Part model, mm, in its own coordinate system. Give positions to 0.01 mm unless a question says otherwise; leave off trailing zeros. Write each loop counter-clockwise with the first axis right and the second up, starting at its lowest first coordinate (ties: lowest second). Pieces come first, ordered by that corner, then holes.
```python
from build123d import *

# Parameters (mm, degrees)
F3_DEPTH = 13.0048
F4_D     = 15
F5_D     = 12
F6_D     = 27.94


with BuildPart() as f3:
    # F2 (on Top) → F3 (new body)
    with BuildSketch(Plane.XY):
        Polygon((54.3151245746, -38.1), (-49.1357887106, -38.1), (-124.5434206745, -187.848847558), (109.6256415023, -187.848847558), align=None)
    extrude(amount=F3_DEPTH)

    # F4 (through all)
    with Locations(Plane(origin=(0, 0, 0), x_dir=(1, 0, 0), z_dir=(0, 0, -1))):
        with Locations((38.4657377694, 60.85), (10.3239816143, 71.2443042339), (27.6568138595, 118.1715758959), (55.7985700146, 107.777271662), (44.9896461047, 165.098847558), (73.1314022598, 154.7045433241)):
            Hole(F4_D / 2)

    # F5 (through all)
    with Locations(Plane(origin=(0, 0, 0), x_dir=(1, 0, 0), z_dir=(0, 0, -1))):
        with Locations((-19.7833501507, 63.7446313346), (-39.4326827285, 53.85), (-66.7141442955, 108.0271081117), (-47.0648117177, 117.9217394463), (-74.3462732846, 172.098847558), (-93.9956058624, 162.2042162234), (-12.8873561721, 170.4100188799)):
            Hole(F5_D / 2)

    # F6 (through all)
    with Locations(Plane(origin=(0, 0, 0), x_dir=(1, 0, 0), z_dir=(0, 0, -1))):
        with Locations((-12.8873561721, 96.8135188799)):
            Hole(F6_D / 2)


solid = f3.part
```
1) Saw through at A-A, the plane x = 76. Write the cut outline in (y, z), then the cut area to 3 significant figures.
Answers follow:
outline: (-187.85, 0) - (-161.63, 0) - (-161.63, 13) - (-187.85, 13) - close; (-147.77, 0) - (-96.81, 0) - (-96.81, 13) - (-147.77, 13) - close
area: 1,000 mm2
2) Saw through at D-D, the plane y = -143. Write the cut outline in (x, z).
Answers follow:
outline: (-101.96, 0) - (93.06, 0) - (93.06, 13) - (-101.96, 13) - close
3) Wall check: L1, parallel to X at y = -170, z = 2; L2, parallel to X at y = -163.5, z = 12.5; L3, parallel to X at y = -105, z = 8.75. Give the ranges that are in metal, low to high.
Answers follow:
L1: x = -115.56 to -79.97, -68.73 to -18.87, -6.9 to 39.31, 50.67 to 103.03
L2: x = -112.28 to -99.85, -88.14 to 37.66, 52.32 to 100.63
L3: x = -82.82 to -71.89, -61.53 to -24.21, -1.57 to 48.83, 62.77 to 79.02
4) Saw through at C-C, the plane x = -23.5. Write the cut outline in (y, z).
Answers follow:
outline: (-187.85, 0) - (-105.9, 0) - (-105.9, 13) - (-187.85, 13) - close; (-87.73, 0) - (-68.45, 0) - (-68.45, 13) - (-87.73, 13) - close; (-59.03, 0) - (-38.1, 0) - (-38.1, 13) - (-59.03, 13) - close
5) Two-plate mould, pull along X, no slides. Class faces 1 (the face through (82.358, -114.023, 6.411)), 2 (the face through (-34.67, -50.2, 6.59)), 3 (the face through (-9, -187.849, 6)): +X half, -X half, draft (parallel to the pull), parting line (faces both ways), or undercut.
Answers follow:
face 1: +X half
face 2: undercut
face 3: draft
6) Pin check, flat tips, straight feed: pin 1 Ø15.5 at (x, y) = (-12.89, -170.41) entering from -Z; pin 2 Ø5 at (y, z) = (-133.5, 6.5) entering from -X; pin 3 Ø4 at (y, z) = (-87.5, 4.5) entering from -X; pin 4 Ø1 at (y, z) = (-81.5, 5) entering from +X. Stop position of each tip, or through.
Answers follow:
pin 1: stops at z = 0
pin 2: stops at x = -98.43
pin 3: stops at x = -75.02
pin 4: stops at x = 70.53
7) Saw through at B-B, the plane z = 9.75. Count the separate pieces of the cut face and the enclosed holes in it, then the cut area to 3 significant figures.
Answers follow:
separate pieces: 1
enclosed holes: 14
area: 22,800 mm2
